The drawing under review shows one solid part. Ordinate dimensions are in mm from its lowest x, y, z. A direction names the side the tool comes from. Coordinates: 2 decimals unless noted, no trailing zeros. Order: outer loops, then holes, each group sorted by start corner. A loop starts at its lowest first (then second) coordinate and runs counter-clockwise, first axis right, second up. Notation, with made-up numbers: (75, 13.25) -> (112, 13.25) arc R14 cw to (112, 31.25) -> close; hole circle Ø4 at (-10.75, 45). An arc over 180 degrees is marked (long way). Use one line per item in the form item = value.
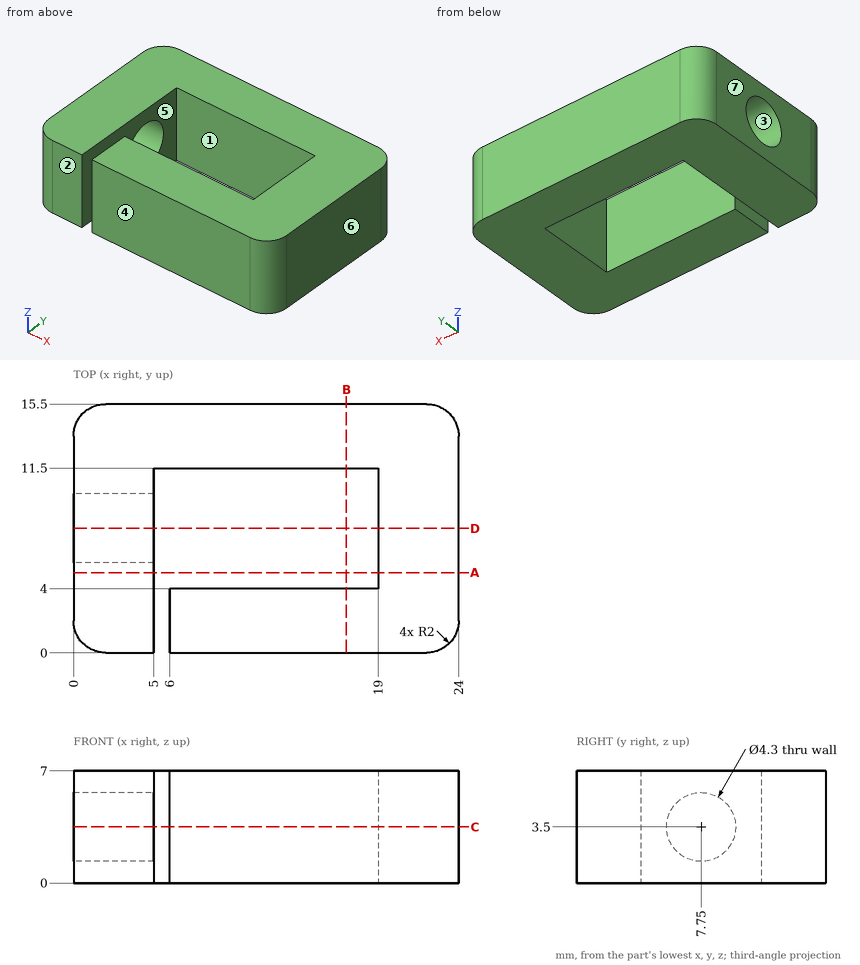
Item 1: To check wall thickness, follow L1, parallel to X at y = 10, z = 0.5; L2, parallel to Y at x = 3.3, z = 3.5; L3, parallel to Y at x = 7, z = 5.5. State the ranges of each line that lie inside material, in increasing order. Write a range as from..to.
Results found:
L1 = 0..5, 19..24
L2 = 0..5.6, 9.9..15.5
L3 = 0..4, 11.5..15.5
Item 2: We need section B-B (x = 17). Write out the cut boundary in (y, z), plus the area to 3 significant figures.
Results found:
outline = (0, 0) -> (4, 0) -> (4, 7) -> (0, 7) -> close; (11.5, 0) -> (15.5, 0) -> (15.5, 7) -> (11.5, 7) -> close
area = 56.0 mm²
Item 3: We need section D-D (y = 7.75). Write out the cut boundary in (x, z).
Results found:
outline = (0, 0) -> (5, 0) -> (5, 1.35) -> (0, 1.35) -> close; (0, 5.65) -> (5, 5.65) -> (5, 7) -> (0, 7) -> close; (19, 0) -> (24, 0) -> (24, 7) -> (19, 7) -> close
Item 4: Tool access review of the marked faces 1, 2 and 3: name each direction out of +Z, -Z, +X, -X, +Y, -Y from which nothing blocks a thin tool from reaching the whole face with its end or side.
Results found:
face_1 = +Z, -Z
face_2 = +Z, -Z, +X, -X, -Y
face_3 = -X
Item 5: Draft analysis for pull direction X (two halves, no side actions). For the marked faces 4, 5, 6 and 7, state which applies: released by +X, released by -X, zero draft, split by the parting line, or undercut.
Results found:
face_4 = zero draft
face_5 = undercut
face_6 = released by +X
face_7 = released by -X
Item 6: We need section C-C (z = 3.5). Write out the cut boundary in (x, y).
Results found:
outline = (0, 2) arc R2 ccw to (2, 0) -> (5, 0) -> (5, 5.6) -> (0, 5.6) -> close; (0, 9.9) -> (5, 9.9) -> (5, 11.5) -> (19, 11.5) -> (19, 4) -> (6, 4) -> (6, 0) -> (22, 0) arc R2 ccw to (24, 2) -> (24, 13.5) arc R2 ccw to (22, 15.5) -> (2, 15.5) arc R2 ccw to (0, 13.5) -> close
Item 7: We need section A-A (y = 5). Write out the cut boundary in (x, z), plus the area to 3 significant figures.
Results found:
outline = (0, 0) -> (5, 0) -> (5, 7) -> (0, 7) -> close; (19, 0) -> (24, 0) -> (24, 7) -> (19, 7) -> close
area = 70.0 mm²
Item 8: Clearance check with a flat-ended pin moving along its axis: pin 1 (4 mm diameter, centred on y = 7.75, z = 3.5, fed in from -X). State where the tip first meets the part, or that it passes through.
Results found:
pin_1 = 19
